Job drawing, mm, ordinate dimensions from the low corner. One solid piece. A direction names the side the tool comes from. Give positions to 0.01 mm unless a question says otherwise; leave off trailing zeros. Order: outer loops, then holes, each group sorted by start corner. A loop starts at its lowest first (then second) coordinate and runs counter-clockwise, first axis right, second up.
Item 1: Two-plate mould, pull along X, no slides. Class the marked faces 1, 2 and 3: released by +X, released by -X, zero draft, split by the parting line, or undercut.
Item 2: Flat gauge pin, fed straight in: P1, Ø6, axis at x = 20, y = 3, coming from the -Z side. Where does the tip first touch, or does it go through?
Item 3: Band-saw the part on C-C on x = 20.25. Give the cut face in (y, z), plus the area to 3 significant figures.
Item 4: Band-saw the part on A-A on z = 5. Give the cut face in (x, y), plus the area to 3 significant figures.
Item 5: Wall check: L1, parallel to X at y = 2.75, z = 2; L2, parallel to X at y = 6.25, z = 6.75 (1 decimal); L3, parallel to X at y = 3.5, z = 11.5 (1 decimal). Give the ranges that are in metal, low to high.
Item 6: Which spindle directions (+Z, -Z, +X, -X, +Y, -Y) get a long thin tool onto all of the face, cutting with end or side? Do the marked faces 4 and 5. Say none if no direction does.
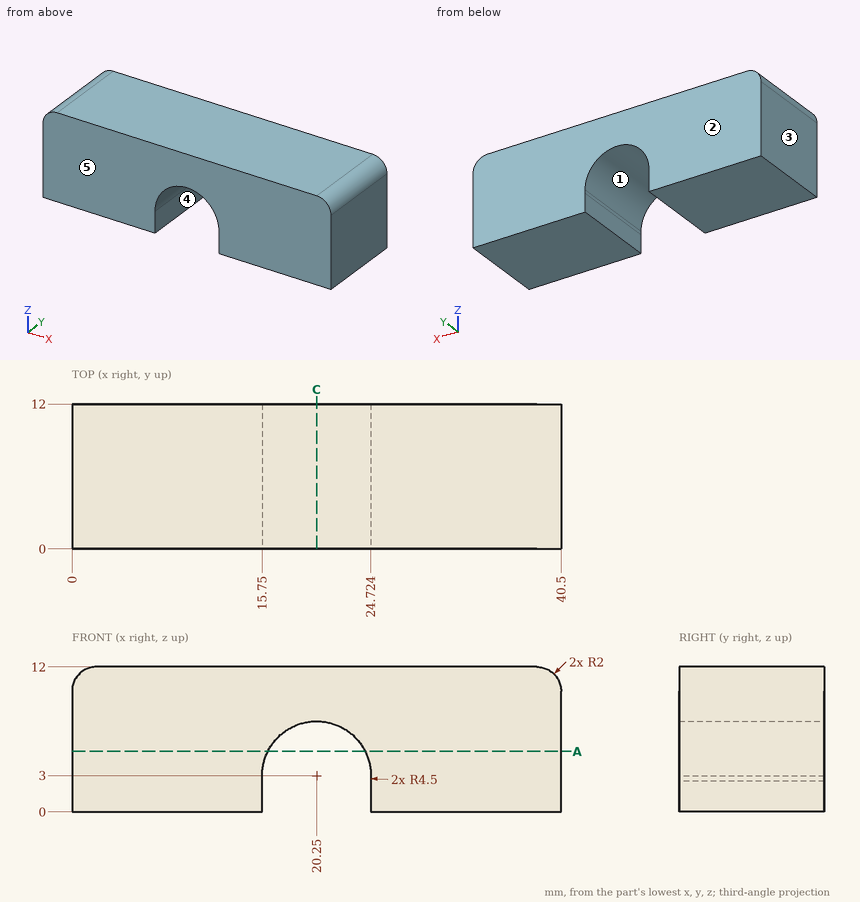
The answers:
1. face 1: undercut
1. face 2: zero draft
1. face 3: released by -X
2. P1: stops at z = 6.11
3. outline: (0, 7.5) - (12, 7.5) - (12, 12) - (0, 12) - close
3. area: 54.0 mm2
4. outline: (0, 0) - (16.22, 0) - (16.22, 12) - (0, 12) - close; (24.28, 0) - (40.5, 0) - (40.5, 12) - (24.28, 12) - close
4. area: 389 mm2
5. L1: x = 0 to 15.75, 24.72 to 40.5
5. L2: x = 0 to 17.8, 22.7 to 40.5
5. L3: x = 0.7 to 39.8
6. face 4: -Z, +Y, -Y
6. face 5: +Z, -Z, +X, -X, -Y
